Check sheet for the modelled part. Datum: model origin and axes. Units: mm. Round coordinates to 2 decimals unless told otherwise and drop trailing zeros. Loops run counter-clockwise (first coordinate to the right, second up) from the corner with the lowest first, then second, coordinate; pieces in that order, holes last. Notation, with made-up numbers: M 65,-38 L 103,-38 A14 ccw 103,-34 Z; hole C -26.5,43.25 d2. An arc over 180 degrees is marked long. Write item = value, one per line. Start each with the question number.
(1) Cross-section at A-A on y = 65. Record the boundary of the cut face in (x, z).
(2) Cross-section at C-C on y = 155. Record the boundary of the cut face in (x, z).
(3) Cross-section at D-D on x = 29. Record the boundary of the cut face in (y, z).
(4) Scan lines: L1, parallel to X at y = 127.5, z = 0.55; L2, parallel to Y at x = 81, z = 0.5; L3, parallel to X at y = 69.5, z = 0.8. Record each from-to range of solid material in increasing order. Write a range as from..to.
(5) Cross-section at B-B on z = 1. Record the boundary of the cut face in (x, y).
(6) Go/stop test with flat-tipped pins: P1, Ø1, axis at x = -25, z = 1, coming from the +Y side; P2, Ø0.6, axis at x = -64, z = 0.5, coming from the +Y side. Record where each tip stops, or that it passes through.
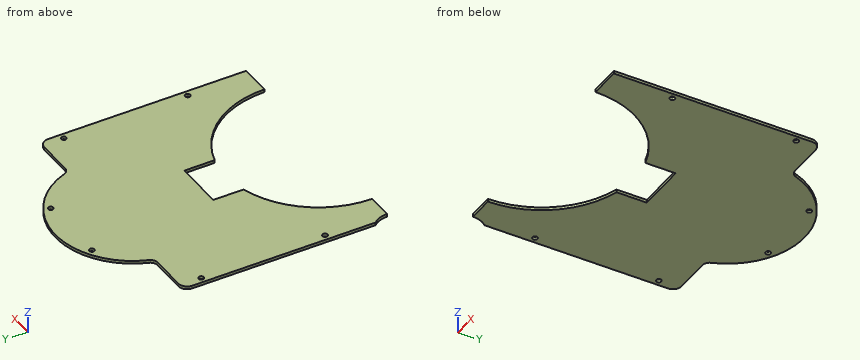
from build123d import *

# Parameters (mm, degrees)
ESQUISSE1_R      = 1.75
EXTRUSION1_DEPTH = 2


with BuildPart() as part:
    # Esquisse1 → Extrusion1 (new body)
    with BuildSketch(Plane.XY):
        with BuildLine():
            Line((79, 142), (54.623712799, 142))
            ThreePointArc((54.623712799, 142), (51.743189619, 142.913120236), (49.914772041, 145.318965517))
            ThreePointArc((49.914772041, 145.318965517), (0, 180.5), (-49.914772041, 145.318965517))
            ThreePointArc((-49.914772041, 145.318965517), (-51.743189619, 142.913120236), (-54.623712799, 142))
            Line((-54.623712799, 142), (-79, 142))
            ThreePointArc((-79, 142), (-83.242640687, 140.242640687), (-85, 136))
            Line((-85, 136), (-85, 10.198039027))
            ThreePointArc((-85, 10.198039027), (-82.035759956, 5.477225575), (-81, 0))
            Line((-81, 0), (-63.5, 0))
            ThreePointArc((-63.5, 0), (-50.555662393, 38.423625545), (-17, 61.182105227))
            Line((-17, 61.182105227), (-17, 82))
            Line((-17, 82), (17, 82))
            Line((17, 82), (17, 61.182105227))
            ThreePointArc((17, 61.182105227), (50.555662393, 38.423625545), (63.5, 0))
            Line((63.5, 0), (85, 0))
            Line((85, 0), (85, 136))
            ThreePointArc((85, 136), (83.242640687, 140.242640687), (79, 142))
        make_face()
        with Locations((-81, 42.5)):
            Circle(ESQUISSE1_R, mode=Mode.SUBTRACT)
        with Locations((-81, 127.5)):
            Circle(ESQUISSE1_R, mode=Mode.SUBTRACT)
        with Locations((-24.25, 169.502232084)):
            Circle(ESQUISSE1_R, mode=Mode.SUBTRACT)
        with Locations(Location((24.25, 169.502232084, 0), (0, 0, 180))):
            Circle(ESQUISSE1_R, mode=Mode.SUBTRACT)
        with Locations(Location((81, 127.5, 0), (0, 0, 180))):
            Circle(ESQUISSE1_R, mode=Mode.SUBTRACT)
        with Locations(Location((81, 42.5, 0), (0, 0, 180))):
            Circle(ESQUISSE1_R, mode=Mode.SUBTRACT)
    extrude(amount=EXTRUSION1_DEPTH)


solid = part.part
Result:
q1.outline = M -85,0 L -17,0 L -17,2 L -85,2 Z; M 17,0 L 85,0 L 85,2 L 17,2 Z
q2.outline = M -45.31,0 L 45.31,0 L 45.31,2 L -45.31,2 Z
q3.outline = M 56.49,0 L 171.86,0 L 171.86,2 L 56.49,2 Z
q4.L1 = -85..-82.75, -79.25..79.25, 82.75..85
q4.L2 = 0..40.75, 44.25..125.75, 129.25..141.66
q4.L3 = -85..-17, 17..85
q5.outline = M -85,10.2 A15 cw -81,0 L -63.5,0 A63.5 cw -17,61.18 L -17,82 L 17,82 L 17,61.18 A63.5 cw 63.5,0 L 85,0 L 85,136 A6 ccw 79,142 L 54.62,142 A5 cw 49.91,145.32 A53 ccw -49.91,145.32 A5 cw -54.62,142 L -79,142 A6 ccw -85,136 Z; hole C -81,42.5 d3.5; hole C -81,127.5 d3.5; hole C -24.25,169.5 d3.5; hole C 24.25,169.5 d3.5; hole C 81,42.5 d3.5; hole C 81,127.5 d3.5
q6.P1 = 174.5
q6.P2 = 142
